Can you work these out from the drawing? Everything is in mm from the part's minimum corner. A direction names the side the tool comes from. Coordinates: 2 decimals unless noted, no trailing zeros. Write each loop counter-clockwise with the first axis right and the second up, starting at its lowest first coordinate (ties: lowest second). Pieces come first, ordered by that corner, then holes.
(1) Imagine slicing it at C-C, the plane x = 22.5. List the corners of the cut face in (y, z) for me (3 decimals).
(2) For pin 1 Ø8 at (x, z) = (8.5, 8) entering from +Y; pin 2 Ø1 at (y, z) = (6.5, 14.5) entering from -X, each with a flat end and sliding along its axis, tell me the tip position at first contact or that it passes through.
(3) Imagine slicing it at D-D, the plane z = 7.75. List the corners of the cut face in (x, y) for me.
(4) Which directions (+Z, -Z, +X, -X, +Y, -Y) give clear straight access to the entire face, cutting with the end or side of a thin tool? Please do the marked faces 5 and 6.
(5) Imagine slicing it at B-B, the plane x = 27. List the corners of the cut face in (y, z) for me, plus the area to 3 significant figures.
(6) Imagine slicing it at A-A, the plane y = 6.75. List the corners of the cut face in (x, z) for me (3 decimals).
(7) Please list where these lines run through material, in increasing order: probe 1 along Y at (x, z) = (22.5, 14.8) (3 decimals); probe 2 along Z at (x, y) = (14.5, 2.5); probe 3 along X at (y, z) = (3.75, 2.5).
(8) Thinking about a two-plate mould opening in Z: for the marked faces 1, 2, 3 and 4, which applies, released by +Z, released by -Z, zero draft, split by the parting line, or undercut?
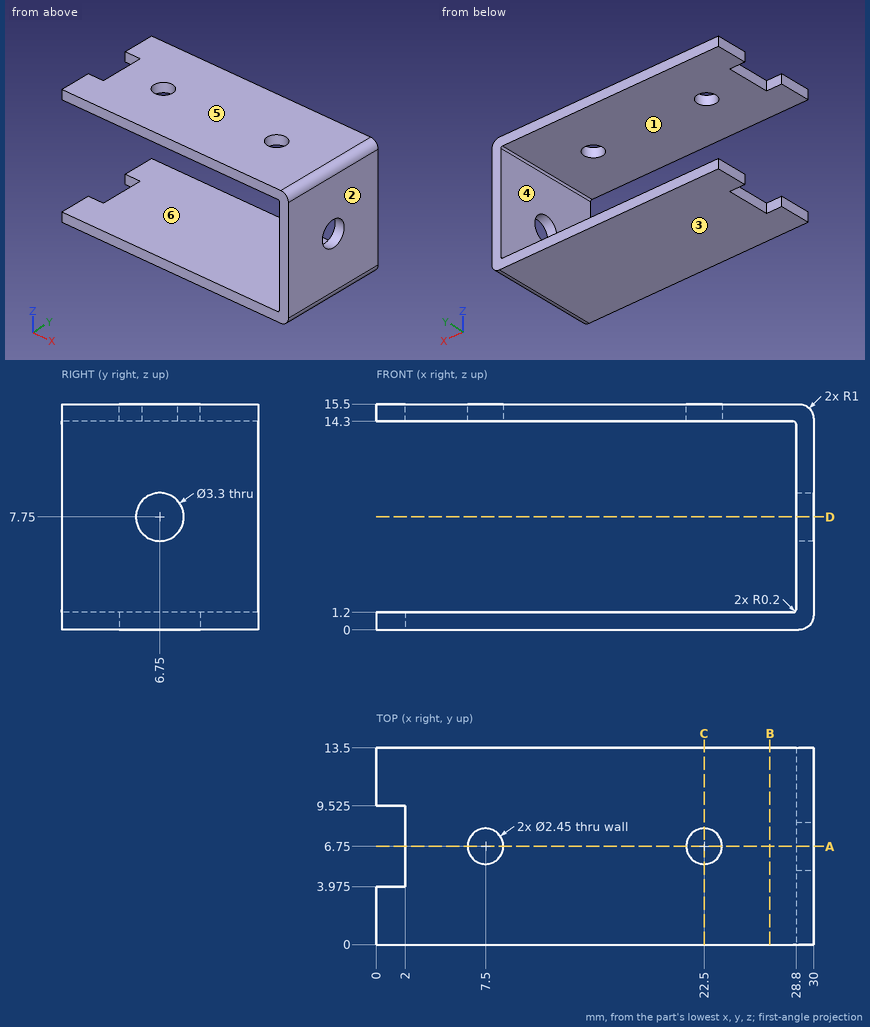
Recorded:
1. outline: (0, 0) - (13.5, 0) - (13.5, 1.2) - (0, 1.2) - close; (0, 14.3) - (5.525, 14.3) - (5.525, 15.5) - (0, 15.5) - close; (7.975, 14.3) - (13.5, 14.3) - (13.5, 15.5) - (7.975, 15.5) - close
2. pin 1: passes through
2. pin 2: stops at x = 2
3. outline: (28.8, 0) - (30, 0) - (30, 5.1) - (28.8, 5.1) - close; (28.8, 8.4) - (30, 8.4) - (30, 13.5) - (28.8, 13.5) - close
4. face 5: +Z, +X, -X, +Y, -Y
4. face 6: -X, +Y, -Y
5. outline: (0, 0) - (13.5, 0) - (13.5, 1.2) - (0, 1.2) - close; (0, 14.3) - (13.5, 14.3) - (13.5, 15.5) - (0, 15.5) - close
5. area: 32.4 mm2
6. outline: (2, 0) - (29, 0) arc R1 ccw to (30, 1) - (30, 6.1) - (28.8, 6.1) - (28.8, 1.4) arc R0.2 cw to (28.6, 1.2) - (2, 1.2) - close; (2, 14.3) - (6.275, 14.3) - (6.275, 15.5) - (2, 15.5) - close; (8.725, 14.3) - (21.275, 14.3) - (21.275, 15.5) - (8.725, 15.5) - close; (23.725, 14.3) - (28.6, 14.3) arc R0.2 cw to (28.8, 14.1) - (28.8, 9.4) - (30, 9.4) - (30, 14.5) arc R1 ccw to (29, 15.5) - (23.725, 15.5) - close
7. probe 1: y = 0 to 5.525, 7.975 to 13.5
7. probe 2: z = 0 to 1.2, 14.3 to 15.5
7. probe 3: x = 28.8 to 30
8. face 1: undercut
8. face 2: zero draft
8. face 3: released by -Z
8. face 4: undercut
